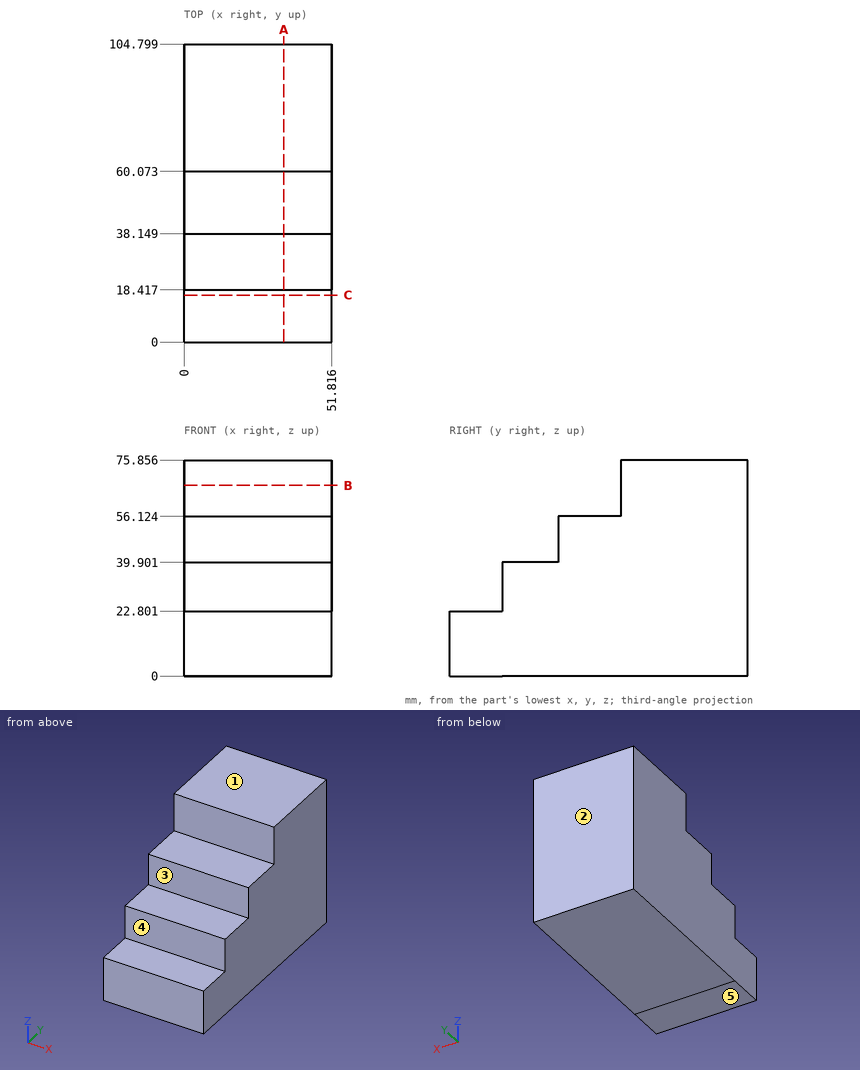
Answer from the drawing. Dimensions are ordinates in mm from the lowest x, y and z of the part. A direction names the side the tool comes from. Round coordinates to 2 decimals unless told otherwise and drop trailing zeros. Order: outer loops, then holes, each group sorted by start corner. A loop starts at its lowest first (then second) coordinate and runs counter-clockwise, first axis right, second up. Notation, with made-up numbers: (-15, 79.25) -> (19, 79.25) arc R19 cw to (19, 103.25) -> close; hole circle Ø7 at (56, 83.5). An arc over 180 degrees is marked (long way). Answer as CSV lines item,"result".
Q1. Which of the six approach directions +Z, -Z, +X, -X, +Y, -Y give full straight-line access (tool end or side, diameter ignored) to the marked faces 4 and 5?
Computed values:
face 4,"+Z, +X, -X, -Y"
face 5,"-Z, +X, -X, +Y, -Y"
Q2. Consider line 1 (Y direction, x = 13, z = 58.5); line 2 (Y direction, x = 6, z = 34); line 3 (Z direction, x = 50.5, y = 19). Determine where each line is inside the solid, lowest interval first. Write a range as from..to.
Computed values:
line 1,"y = 60.07..104.8"
line 2,"y = 18.42..104.8"
line 3,"z = 0..39.9"
Q3. A cutting plane is placed at B-B on z = 67. Determine the outline of the cut face in (x, y), plus the area to 3 significant figures.
Computed values:
outline,"(0, 60.07) -> (51.82, 60.07) -> (51.82, 104.8) -> (0, 104.8) -> close"
area,"2,320 mm^2"
Q4. Given pin 1 (24 mm diameter, centred on x = 34.5, y = 45.5, fed in from +Z); pin 2 (21.5 mm diameter, centred on x = 19, z = 67.5, fed in from -Y); pin 3 (20.5 mm diameter, centred on x = 32.5, y = 8, fed in from +Z), each flat-ended and moving along its own axis, determine where each tip first touches the part or whether it passes through.
Computed values:
pin 1,"stops at z = 56.12"
pin 2,"stops at y = 60.07"
pin 3,"stops at z = 22.8"
Q5. For a pull along Y with two mould halves and no side action, classify the marked faces 1, 2 and 3 as +Y half, -Y half, draft (parallel to the pull), parting line (faces both ways), or undercut.
Computed values:
face 1,"draft"
face 2,"+Y half"
face 3,"-Y half"
Q6. A cutting plane is placed at C-C on y = 16.5. Determine the outline of the cut face in (x, z), plus the area to 3 significant figures.
Computed values:
outline,"(0, 0) -> (51.82, 0) -> (51.82, 22.8) -> (0, 22.8) -> close"
area,"1,180 mm^2"
Q7. A cutting plane is placed at A-A on x = 35. Determine the outline of the cut face in (y, z) (1 decimal).
Computed values:
outline,"(0, 0) -> (104.8, 0) -> (104.8, 75.9) -> (60.1, 75.9) -> (60.1, 56.1) -> (38.1, 56.1) -> (38.1, 39.9) -> (18.4, 39.9) -> (18.4, 22.8) -> (0, 22.8) -> close"
